from build123d import *

# Parameters (mm, degrees)
SKETCH_1_R      = 4
EXTRUDE_1_DEPTH = 2
SKETCH_2_W      = 40
SKETCH_2_H      = 2
EXTRUDE_2_DEPTH = 20


with BuildPart() as part:
    # 草图1 → 凸台-拉伸1 (new body)
    with BuildSketch(Plane.XY):
        with BuildLine():
            Line((-4.303483184, 8.671520648), (4.196516816, 8.671520648))
            Line((4.196516816, 8.671520648), (74.196516816, 8.671520648))
            Line((74.196516816, 8.671520648), (74.196516816, -8.328479352))
            Line((74.196516816, -8.328479352), (-4.303483184, -8.328479352))
            ThreePointArc((-4.303483184, -8.328479352), (-12.803483184, 0.171520648), (-4.303483184, 8.671520648))
        make_face()
        with Locations((-5.803483184, 0.171520648)):
            Circle(SKETCH_1_R, mode=Mode.SUBTRACT)
    extrude_1 = extrude(amount=EXTRUDE_1_DEPTH)

    # 草图2 → 凸台-拉伸2 (add)
    with BuildSketch(Plane(origin=(0, 0, 0), x_dir=(-1, 0, 0), z_dir=(0, 0, -1))):
        with Locations((-54.196516816, 7.671520648)):
            Rectangle(SKETCH_2_W, SKETCH_2_H)
    extrude(amount=EXTRUDE_2_DEPTH)

    # 镜向1: 凸台-拉伸1 across plane
    add(extrude_1.mirror(Plane(origin=(0, 0, -10), x_dir=(1, 0, 0), z_dir=(0, 0, -1))))


solid = part.part
For this review, take the finished solid that the model builds, in its own axes (mm). A direction names the side the tool comes from. Give positions to 0.01 mm unless a question says otherwise; leave off trailing zeros. Write each loop counter-clockwise with the first axis right and the second up, starting at its lowest first coordinate (ties: lowest second). Pieces come first, ordered by that corner, then holes. Notation, with made-up numbers: (80, -24.75) -> (119, -24.75) arc R26 ccw to (119, -2.75) -> close; hole circle Ø9 at (58.25, 57.5). An arc over 180 degrees is marked (long way). Use CSV: the item, a comma, the result in double quotes.
Q1. Take a section at B-B, the plane y = -1.5. Write out the cut boundary in (x, z).
Conclusion:
outline,"(-12.64, -22) -> (-9.44, -22) -> (-9.44, -20) -> (-12.64, -20) -> close; (-12.64, 0) -> (-9.44, 0) -> (-9.44, 2) -> (-12.64, 2) -> close; (-2.17, -22) -> (74.2, -22) -> (74.2, -20) -> (-2.17, -20) -> close; (-2.17, 0) -> (74.2, 0) -> (74.2, 2) -> (-2.17, 2) -> close"
Q2. For P1, Ø1, axis at y = 8, z = -9.5, coming from the -X side; P2, Ø6.5, axis at x = -5.8, y = 0.17, coming from the +Z side; P3, Ø1.5, axis at y = 3.5, z = -0.5, coming from the -X side; P4, Ø2, axis at x = 45, z = -8.5, coming from the -Y side, all flat-tipped, find the tip position at first contact; note any pin that passes through.
Conclusion:
P1,"x = 34.2"
P2,"through"
P3,"x = -12.34"
P4,"y = 6.67"
Q3. Mouldability with a two-part tool opening along Z and no side actions: class faces 3 (the face through (31, 0, -22)), 4 (the face through (31, 0, 2)), 5 (the face through (-8.98, -2.26, -20.99)), 6 (the face through (54, 6.672, -10)) as pulls with the +Z half, pulls with the -Z half, needs draft (parallel to the pull), parting line crosses it, or undercut.
Conclusion:
face 3,"pulls with the -Z half"
face 4,"pulls with the +Z half"
face 5,"needs draft"
face 6,"undercut"
Q4. Take a section at D-D, the plane x = 66.5. Write out the cut boundary in (y, z).
Conclusion:
outline,"(-8.33, -22) -> (8.67, -22) -> (8.67, 2) -> (-8.33, 2) -> (-8.33, 0) -> (6.67, 0) -> (6.67, -20) -> (-8.33, -20) -> close"
Q5. Take a section at C-C, the plane y = -6.75. Write out the cut boundary in (x, z).
Conclusion:
outline,"(-9.24, -22) -> (74.2, -22) -> (74.2, -20) -> (-9.24, -20) -> close; (-9.24, 0) -> (74.2, 0) -> (74.2, 2) -> (-9.24, 2) -> close"
Q6. Take a section at A-A, the plane x = 9. Write out the cut boundary in (y, z), then the cut area to 3 significant figures.
Conclusion:
outline,"(-8.33, -22) -> (8.67, -22) -> (8.67, -20) -> (-8.33, -20) -> close; (-8.33, 0) -> (8.67, 0) -> (8.67, 2) -> (-8.33, 2) -> close"
area,"68.0 mm2"
Q7. To check wall thickness, follow probe 1 along Z at (x, y) = (4, 7.75); probe 2 along Y at (x, z) = (66, -19.75); probe 3 along X at (y, z) = (7.75, -17.25). State the ranges of each line that lie inside material, in increasing order. Write a range as [from, to].
Conclusion:
probe 1,"[-22, -20], [0, 2]"
probe 2,"[6.67, 8.67]"
probe 3,"[34.2, 74.2]"
Q8. Tool access review of faces 1 (the face through (34.197, 8, -10)), 2 (the face through (43, 8.672, -10)): name each direction out of +Z, -Z, +X, -X, +Y, -Y from which nothing blocks a thin tool from reaching the whole face with its end or side.
Conclusion:
face 1,"-X, +Y, -Y"
face 2,"+Z, -Z, +X, -X, +Y"
